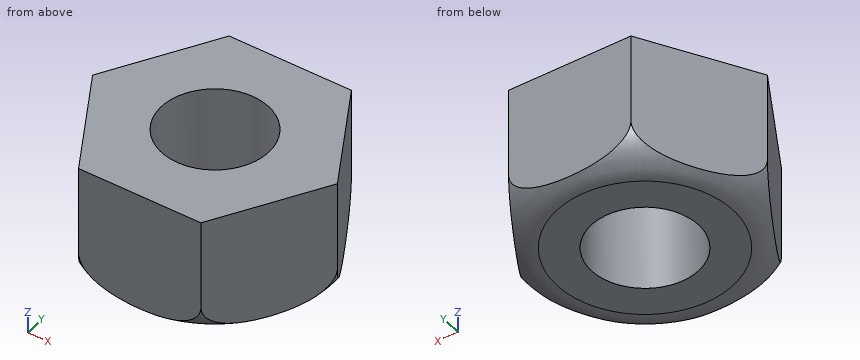
```python
from build123d import *

# Parameters (mm, degrees)
BOSS_EXTRUDE1_DEPTH = 35
SKETCH2_R           = 15
CUT_EXTRUDE1_DEPTH  = 35


with BuildPart() as part:
    # Sketch1 → Boss-Extrude1 (new body)
    with BuildSketch(Plane.XY):
        Polygon((-34.641016151, 0), (-17.320508076, -30), (17.320508076, -30), (34.641016151, 0), (17.320508076, 30), (-17.320508076, 30), align=None)
    extrude(amount=BOSS_EXTRUDE1_DEPTH)

    # Sketch2 → Cut-Extrude1 (cut)
    with BuildSketch(Plane.XY.offset(35)):
        Circle(SKETCH2_R)
    extrude(amount=-CUT_EXTRUDE1_DEPTH, mode=Mode.SUBTRACT)

    # Sketch3 → Cut-Revolve1 (revolve, cut)
    with BuildSketch(Plane(origin=(0, 0, 0), x_dir=(1, 0, 0), z_dir=(0, 1, 0))):
        with BuildLine():
            Line((24.641016151, 0), (34.641016151, 0))
            Line((34.641016151, 0), (34.641016151, -10))
            ThreePointArc((34.641016151, -10), (31.712083963, -2.928932188), (24.641016151, 0))
        make_face()
    revolve(axis=Axis((0, 0, 0), (0, 0, 1)), mode=Mode.SUBTRACT)


solid = part.part
```
The listing builds one solid part. Answer for the finished solid, in the listing's coordinates (mm). Give positions to 0.01 mm unless a question says otherwise; leave off trailing zeros. Order: outer loops, then holes, each group sorted by start corner. A loop starts at its lowest first (then second) coordinate and runs counter-clockwise, first axis right, second up. Notation, with made-up numbers: (81, 45) - (120, 45) arc R34 ccw to (120, 83) - close; hole circle Ø5 at (63, -16.5). An arc over 180 degrees is marked (long way). Answer in a Markdown table with one row per item. Add a question column.
Q1. Given P1, Ø5, axis at y = 24, z = 12.5, coming from the -X side; P2, Ø1.5, axis at y = -14, z = 22, coming from the +X side; P3, Ø6, axis at x = -4, y = -10.5, coming from the -Z side; P4, Ø1.5, axis at y = -20, z = 20.5, coming from the +X side, each flat-ended and moving along its own axis, determine where each tip first touches the part or whether it passes through.
Q2. Find the intervals of material crossed by line 1 along Y through (x, z) = (0, 14); line 2 along X through (y, z) = (-8, 22); line 3 along X through (y, z) = (13, 12), in increasing order. Write a range as [from, to].
Q3. The part is cut by section B-B (x = 0). Determine the outline of the cut face in (y, z), then the cut area to 3 significant figures.
Q4. The part is cut by section A-A (z = 27). Determine the outline of the cut face in (x, y), then the cut area to 3 significant figures.
Q5. The part is cut by section C-C (z = 9). Determine the outline of the cut face in (x, y), then the cut area to 3 significant figures.
Q6. The part is cut by section D-D (z = 4.5). Determine the outline of the cut face in (x, y), then the cut area to 3 significant figures.
Determined:
| question | item | result |
|---|---|---|
| 1 | P1 | stops at x = -22.23 |
| 1 | P2 | stops at x = 26.99 |
| 1 | P3 | passes through |
| 1 | P4 | stops at x = 23.53 |
| 2 | line 1 | y = [-30, -15], [15, 30] |
| 2 | line 2 | x = [-30.02, -12.69], [12.69, 30.02] |
| 2 | line 3 | x = [-27.14, -7.48], [7.48, 27.14] |
| 3 | outline | (-30, 1.56) arc R10 ccw to (-24.64, 0) - (-15, 0) - (-15, 35) - (-30, 35) - close; (15, 0) - (24.64, 0) arc R10 ccw to (30, 1.56) - (30, 35) - (15, 35) - close |
| 3 | area | 1,040 mm² |
| 4 | outline | (-34.64, 0) - (-17.32, -30) - (17.32, -30) - (34.64, 0) - (17.32, 30) - (-17.32, 30) - close; hole circle Ø30 at (0, 0) |
| 4 | area | 2,410 mm² |
| 5 | outline | (-34.59, -0.09) - (-17.37, -29.91) arc R34.59 ccw to (-17.22, -30) - (17.22, -30) arc R34.59 ccw to (17.37, -29.91) - (34.59, -0.09) arc R34.59 ccw to (34.59, 0.09) - (17.37, 29.91) arc R34.59 ccw to (17.22, 30) - (-17.22, 30) arc R34.59 ccw to (-17.37, 29.91) - (-34.59, 0.09) arc R34.59 ccw to start; hole circle Ø30 at (0, 0) |
| 5 | area | 2,410 mm² |
| 6 | outline | (-32.85, -3.11) - (-19.12, -26.89) arc R32.99 ccw to (-13.73, -30) - (13.73, -30) arc R32.99 ccw to (19.12, -26.89) - (32.85, -3.11) arc R32.99 ccw to (32.85, 3.11) - (19.12, 26.89) arc R32.99 ccw to (13.73, 30) - (-13.73, 30) arc R32.99 ccw to (-19.12, 26.89) - (-32.85, 3.11) arc R32.99 ccw to start; hole circle Ø30 at (0, 0) |
| 6 | area | 2,380 mm² |
